```python
from build123d import *

# Parameters (mm, degrees)
F0_W     = 20
F0_H     = 40
F1_DEPTH = 690
F3_D     = 5
F3_DEPTH = 20
F3_TIP   = 1.5021515476
F4_W     = 20
F4_H     = 20
F5_DEPTH = 66.8
F6_W     = 20
F6_H     = 20
F7_DEPTH = 25


with BuildPart() as f1:
    # F0 (on Top) → F1 (new body)
    with BuildSketch(Plane.XY):
        Rectangle(F0_W, F0_H)
    extrude(amount=F1_DEPTH)

    # F3
    with Locations(Plane(origin=(0, 20, 0), x_dir=(-1, 0, 0), z_dir=(0, 1, 0))):
        with Locations((0, 570), (0, 420), (0, 270), (0, 120)):
            Hole(F3_D / 2, depth=F3_DEPTH)
            with Locations((0, 0, -(F3_DEPTH + F3_TIP / 2))):  # 118° drill point
                Cone(0, F3_D / 2, F3_TIP, mode=Mode.SUBTRACT)

    # F4 (on face) → F5 (cut)
    with BuildSketch(Plane.YZ.offset(10)):
        with Locations((0, 680)):
            Rectangle(F4_W, F4_H)
    extrude(amount=-F5_DEPTH, mode=Mode.SUBTRACT)

    # F6 (on face) → F7 (cut)
    with BuildSketch(Plane.YZ.offset(10)):
        with Locations((0, 10)):
            Rectangle(F6_W, F6_H)
    extrude(amount=-F7_DEPTH, mode=Mode.SUBTRACT)


with BuildPart() as f8_1:
    # F8: copy of F1
    add(f1.part)


solid = f1.part
```
Model file for the job. Use its own axes, mm. A direction names the side the tool comes from. Coordinates: 2 decimals unless noted, no trailing zeros. Order: outer loops, then holes, each group sorted by start corner. A loop starts at its lowest first (then second) coordinate and runs counter-clockwise, first axis right, second up. Notation, with made-up numbers: (63, 56) - (82, 56) arc R19 ccw to (82, 72) - close; hole circle Ø8 at (-18.75, 11.25). An arc over 180 degrees is marked (long way). Return JSON: item names as keys, results as strings. Group by question number.
1) Tool access for faces 1 (the flat face through (-10, 0, 340)), 2 (the flat face through (0, 10, 680)), 3 (the flat face through (0, -10, 10)): list every direction of +Z, -Z, +X, -X, +Y, -Y with a clear straight run to the whole face (end or side of a thin tool).
2) Saw through at A-A, the plane x = 5.5. Write the cut outline in (y, z), plus the area to 3 significant figures.
3) Flat gauge pins, fed straight in: P1, Ø5, axis at x = -6, y = 0.5, coming from the -Z side; P2, Ø1.5, axis at x = -1, y = 3.5, coming from the +Z side. Where does each tip first touch, or does it go through?
4) Mould opens along Y. For faces 4 (the flat face through (10, 0, 340)), 5 (the flat face through (0, 10, 10)), 6 (the flat face through (0, 20, 340)), 7 (the flat face through (0, 0, 20)) say: released by +Y, released by -Y, zero draft, split by the parting line, or undercut.
5) Probe line 1 (Z direction, x = 0, y = 4.5); line 2 (Z direction, x = 0, y = 13); line 3 (X direction, y = 14.75, z = 270). List the from-to ranges inside material, lowest first. Write a range as from..to.
Values found:
{
 "1": {"face 1": "+Z, -Z, -X, +Y, -Y", "face 2": "+Z, +X, -X", "face 3": "-Z, +X, -X"},
 "2": {"outline": "(-20, 0) - (-10, 0) - (-10, 20) - (10, 20) - (10, 0) - (20, 0) - (20, 690) - (10, 690) - (10, 670) - (-10, 670) - (-10, 690) - (-20, 690) - close", "area": "26,800 mm²"},
 "3": {"P1": "stops at z = 20", "P2": "stops at z = 670"},
 "4": {"face 4": "zero draft", "face 5": "undercut", "face 6": "released by +Y", "face 7": "undercut"},
 "5": {"line 1": "z = 20..117.5, 122.5..267.5, 272.5..417.5, 422.5..567.5, 572.5..670", "line 2": "z = 0..117.5, 122.5..267.5, 272.5..417.5, 422.5..567.5, 572.5..690", "line 3": "x = -10..-2.5, 2.5..10"}
}
